Job drawing, mm, ordinate dimensions from the low corner. One solid piece. Give positions to 0.01 mm unless a question says otherwise; leave off trailing zeros. Loops run counter-clockwise (first coordinate to the right, second up) from the corner with the lowest first, then second, coordinate; pieces in that order, holes last. Notation, with made-up numbers: (71.25, -21.5) -> (80.25, -21.5) arc R18 ccw to (80.25, -16.5) -> close; hole circle Ø9 at (17, 54). An arc over 180 degrees is marked (long way). Answer as a JSON object with one key per item and string values. Group by question number.
Q1. Band-saw the part on B-B, the plane y = 3.5. Write the cut outline in (x, z) (3 decimals).
Q2. Band-saw the part on A-A, the plane x = 5. Write the cut outline in (y, z) (3 decimals), plus the area to 3 significant figures.
Q3. Wall check: probe 1 along Y at (x, z) = (5, 0.5) (3 decimals); probe 2 along X at (y, z) = (3, 2.35). Give the ranges that are in metal, low to high. Write a range as from..to.
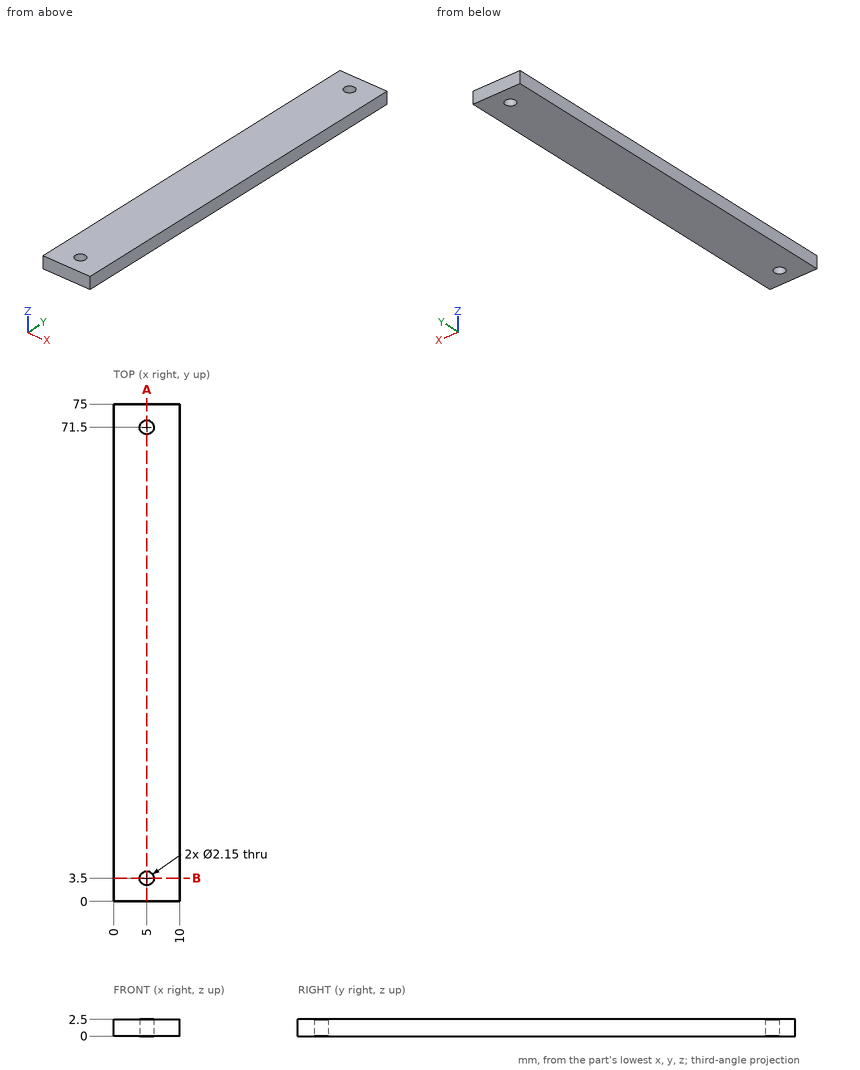
Worked answers:
{
 "1": {"outline": "(0, 0) -> (3.925, 0) -> (3.925, 2.5) -> (0, 2.5) -> close; (6.075, 0) -> (10, 0) -> (10, 2.5) -> (6.075, 2.5) -> close"},
 "2": {"outline": "(0, 0) -> (2.425, 0) -> (2.425, 2.5) -> (0, 2.5) -> close; (4.575, 0) -> (70.425, 0) -> (70.425, 2.5) -> (4.575, 2.5) -> close; (72.575, 0) -> (75, 0) -> (75, 2.5) -> (72.575, 2.5) -> close", "area": "177 mm2"},
 "3": {"probe 1": "0..2.425, 4.575..70.425, 72.575..75", "probe 2": "0..4.05, 5.95..10"}
}
